Could you check a few things on this model? Use its own coordinates, in mm. A direction names the side the tool comes from. Give positions to 0.01 mm unless a question says otherwise; leave off trailing zeros. Order: outer loops, then holes, each group sorted by start corner. A loop starts at its lowest first (then second) coordinate and runs counter-clockwise, first axis right, second up.
(1) Imagine slicing it at B-B, the plane z = 7. Write out the boundary of the cut face in (x, y).
(2) On a 3-axis mill with a long thin cutter (end or side, diameter ignored), from which of +Z, -Z, +X, -X, +Y, -Y can I reach the whole of each face in a straight line? I mean faces 1 (the flat face through (64, 5.5, 42)), 2 (the flat face through (58.757, 0, 26)), 3 (the flat face through (-83, 0, 11)), 4 (the cylindrical face through (-26.238, 0.22, 45.463)). Say none if no direction works.
(3) If I drill on probe 1 along X at (y, z) = (-17, 18); probe 2 along X at (y, z) = (-12, 27); probe 3 along X at (y, z) = (2, 2), over which ranges is the centre line in solid material (lowest first)?
(4) Imagine slicing it at C-C, the plane z = 30.5. Write out the boundary of the cut face in (x, y), then the cut area to 3 significant figures.
(5) Imagine slicing it at D-D, the plane x = 41.5. Write out the boundary of the cut face in (y, z).
(6) Imagine slicing it at A-A, the plane y = 10.5. Write out the boundary of the cut face in (x, z), then the cut area to 3 significant figures.
(7) Will these pins go through, and if not, where does the flat tip stop? pin 1 (16 mm diameter, centred on x = -21.24, y = 0, fed in from +Z); pin 2 (5 mm diameter, centred on y = 13.5, z = 41, fed in from -X); pin 3 (8 mm diameter, centred on y = 13, z = 33.5, fed in from -X); pin 4 (4.5 mm diameter, centred on x = -21.24, y = 0, fed in from +Z).
from build123d import *

# Parameters (mm, degrees)
F0_W           = 26
F0_H           = 11
F0_W_2         = 38
F1_DEPTH       = 20.5
F2_R           = 5
F3_R           = 5
F4_R           = 4
F5_DEPTH       = 12
F7_DEPTH       = 25
F9_D           = 5
F9_START       = 4.8890258
F9_CSINK_D     = 10
F9_CSINK_ANGLE = 90


# Not quite as in the source:
# - a feature names something its author has since deleted; it is built from what else it names


with BuildPart() as f1:
    # F0 (on Front) → F1 (new body, symmetric)
    with BuildSketch(Plane.XZ):
        with Locations((-84.2427663654, 5.5)):
            Rectangle(F0_W, F0_H)
        with BuildLine():
            Line((-69.9081892337, 11), (-71.2427663654, 11))
            Line((-71.2427663654, 11), (-71.2427663654, 0))
            ThreePointArc((-71.2427663654, 0), (-70.9079032421, 5.5403315812), (-69.9081892337, 11))
        make_face()
        with BuildLine():
            ThreePointArc((-69.9081892337, 11), (-70.9079032421, 5.5403315812), (-71.2427663654, 0))
            Line((-71.2427663654, 0), (-60.2427663654, 0))
            ThreePointArc((-60.2427663654, 0), (-25.2427663654, 35), (9.7572336346, 0))
            Line((9.7572336346, 0), (20.7572336346, 0))
            ThreePointArc((20.7572336346, 0), (20.4223705113, 5.5403315812), (19.4226565028, 11))
            ThreePointArc((19.4226565028, 11), (-25.2427663654, 46), (-69.9081892337, 11))
        make_face()
        with BuildLine():
            ThreePointArc((19.4226565028, 11), (20.4223705113, 5.5403315812), (20.7572336346, 0))
            Line((20.7572336346, 0), (20.7572336346, 11))
            Line((20.7572336346, 11), (19.4226565028, 11))
        make_face()
        with Locations((39.7572336346, 5.5)):
            Rectangle(F0_W_2, F0_H)
        Polygon((58.7572336346, 11), (58.7572336346, 0), (69.7572336346, 0), (69.7572336346, 50), (58.7572336346, 50), align=None)
    extrude(amount=F1_DEPTH, both=True)

    # F2
    f2_edges = [f1.edges().sort_by_distance(p)[0] for p in [
        (-97.242766, -20.5, 5.5),
        (-97.242766, 20.5, 5.5),
    ]]
    fillet(f2_edges, radius=F2_R)

    # F3
    f3_edges = [f1.edges().sort_by_distance(p)[0] for p in [
        (64.257234, -20.5, 50),
        (64.257234, 20.5, 50),
    ]]
    fillet(f3_edges, radius=F3_R)

    # F4 (on face) → F5 (cut)
    with BuildSketch(Plane.XY.offset(11)):
        with Locations((-87.2427663654, 10.5)):
            Circle(F4_R)
        with Locations((-87.2427663654, -10.5)):
            Circle(F4_R)
    extrude(amount=-F5_DEPTH, mode=Mode.SUBTRACT)

    # F6 (on face) → F7 (cut)
    with BuildSketch(Plane.YZ.offset(69.7572336346)):
        with BuildLine():
            Line((5.5, 50), (-5.5, 50))
            Line((-5.5, 50), (-5.5, 45))
            Line((-5.5, 45), (-5.5, 34))
            ThreePointArc((-5.5, 34), (0, 39.5), (5.5, 34))
            Line((5.5, 34), (5.5, 45))
            Line((5.5, 45), (5.5, 50))
        make_face()
        with BuildLine():
            ThreePointArc((5.5, 34), (0, 39.5), (-5.5, 34))
            Line((-5.5, 34), (5.5, 34))
        make_face()
        with BuildLine():
            Line((5.5, 34), (-5.5, 34))
            ThreePointArc((-5.5, 34), (0, 28.5), (5.5, 34))
        make_face()
    extrude(amount=-F7_DEPTH, mode=Mode.SUBTRACT)

    # F9 (through all)
    # its depths count from where the whole tool has entered the part; down to there all is cleared
    with Locations(Plane.XY.offset(50).offset(-F9_START)):
        with Locations((-21.2427663654, 0)):
            CounterSinkHole(F9_D / 2, F9_CSINK_D / 2, counter_sink_angle=F9_CSINK_ANGLE)


solid = f1.part
Answer block:
1. outline: (-97.24, -15.5) arc R5 ccw to (-92.24, -20.5) - (-59.54, -20.5) - (-59.54, 20.5) - (-92.24, 20.5) arc R5 ccw to (-97.24, 15.5) - close; (9.05, -20.5) - (69.76, -20.5) - (69.76, 20.5) - (9.05, 20.5) - close; hole circle Ø8 at (-87.24, -10.5); hole circle Ø8 at (-87.24, 10.5)
2. face 1: +Z, +X
2. face 2: +Z, +Y, -Y
2. face 3: +Z, -X, +Y, -Y
2. face 4: +Z
3. probe 1: x = -67.57 to -55.26, 4.77 to 17.09, 58.76 to 69.76
3. probe 2: x = -62.49 to -47.51, -2.97 to 12, 58.76 to 69.76
3. probe 3: x = -97.24 to -60.19, 9.7 to 69.76
4. outline: (-59.68, -20.5) - (-42.41, -20.5) - (-42.41, 20.5) - (-59.68, 20.5) - close; (-8.07, -20.5) - (9.19, -20.5) - (9.19, 20.5) - (-8.07, 20.5) - close; (58.76, -20.5) - (69.76, -20.5) - (69.76, -4.24) - (58.76, -4.24) - close; (58.76, 4.24) - (69.76, 4.24) - (69.76, 20.5) - (58.76, 20.5) - close
4. area: 1,770 mm2
5. outline: (-20.5, 0) - (20.5, 0) - (20.5, 11) - (-20.5, 11) - close
6. outline: (-97.24, 0) - (-91.24, 0) - (-91.24, 11) - (-97.24, 11) - close; (-83.24, 0) - (-60.24, 0) arc R35 cw to (9.76, 0) - (69.76, 0) - (69.76, 50) - (58.76, 50) - (58.76, 11) - (19.42, 11) arc R46 ccw to (-69.91, 11) - (-83.24, 11) - close
6. area: 2,580 mm2
7. pin 1: stops at z = 46
7. pin 2: stops at x = -50.42
7. pin 3: stops at x = -60.54
7. pin 4: passes through
